Geometry: see drawing. Coordinates: mm, zero at the bounding-box minimum. Round coordinates to 2 decimals unless told otherwise and drop trailing zeros. Write each loop counter-clockwise with the first axis right and the second up, starting at its lowest first coordinate (ties: lowest second). Pieces come first, ordered by that corner, then holes.
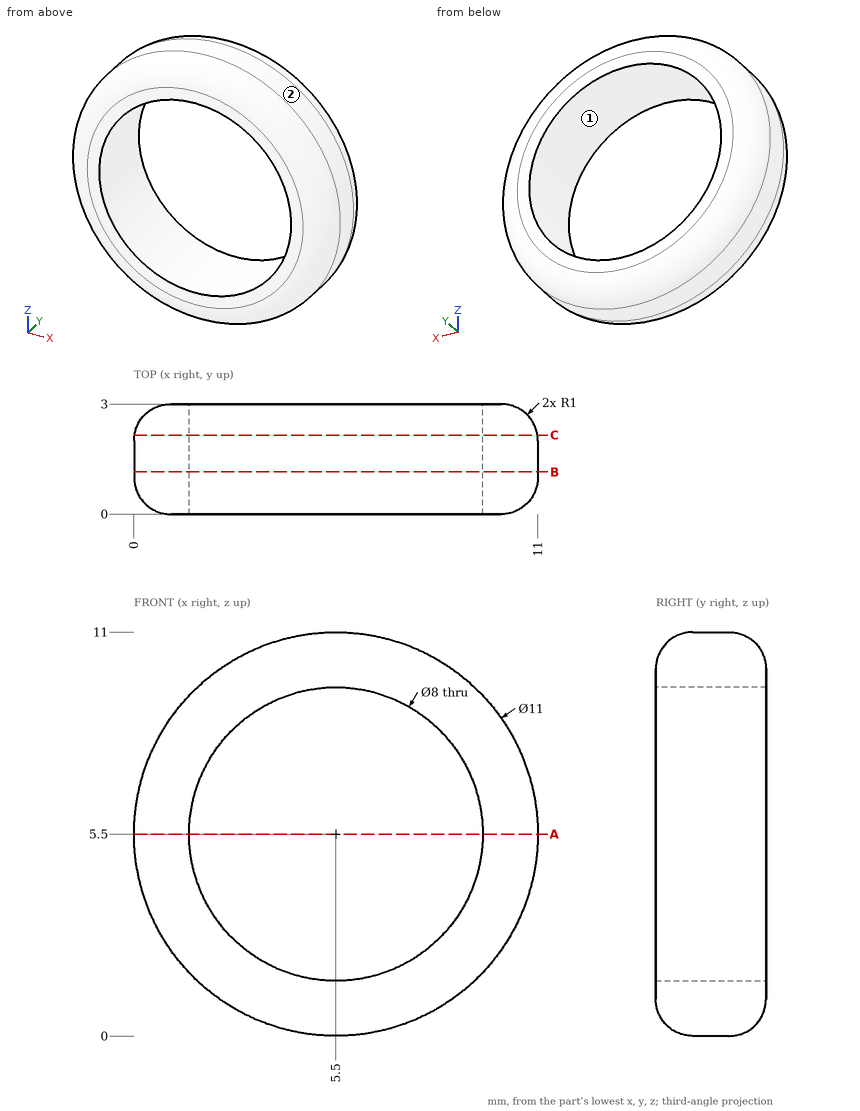
Q1. Section query A-A, the plane z = 5.5. Output: boundary loops of the cut face in (x, y).
Q2. Section query B-B, the plane y = 1.15. Output: boundary loops of the cut face in (x, z).
Q3. Mould query, pull axis Z, two halves, no side actions, for the marked faces 1 and 2. Classes: pulls with the +Z half, pulls with the -Z half, needs draft (parallel to the pull), parting line crosses it, or undercut.
Q4. Section query C-C, the plane y = 2.15. Output: boundary loops of the cut face in (x, z).
Q5. Line query: line 1 (X direction, y = 1.9, z = 5.5); line 2 (X direction, y = 2.7, z = 5.5); line 3 (Z direction, x = 5.75, y = 2.15). Output: solid intervals per line, ascending.
Filled in:
1. outline: (0, 1) arc R1 ccw to (1, 0) - (1.5, 0) - (1.5, 3) - (1, 3) arc R1 ccw to (0, 2) - close; (9.5, 0) - (10, 0) arc R1 ccw to (11, 1) - (11, 2) arc R1 ccw to (10, 3) - (9.5, 3) - close
2. outline: circle Ø11 at (5.5, 5.5); hole circle Ø8 at (5.5, 5.5)
3. face 1: undercut
3. face 2: parting line crosses it
4. outline: circle Ø10.98 at (5.5, 5.5); hole circle Ø8 at (5.5, 5.5)
5. line 1: x = 0 to 1.5, 9.5 to 11
5. line 2: x = 0.29 to 1.5, 9.5 to 10.71
5. line 3: z = 0.02 to 1.51, 9.49 to 10.98
